Here's the drawing with two shaded views (mm, measured from the low corner). I have some questions. A direction names the side the tool comes from. Give positions to 0.01 mm unless a question says otherwise; leave off trailing zeros. Loops run counter-clockwise (first coordinate to the right, second up) from the corner with the lowest first, then second, coordinate; pieces in that order, holes last. Notation, with made-up numbers: (-32.5, 12.25) - (22.5, 12.25) arc R18 ccw to (22.5, 28.25) - close; hole circle Ø8 at (-33.5, -24). An arc over 180 degrees is marked (long way). Use a Markdown table: item, result. Add a question column.
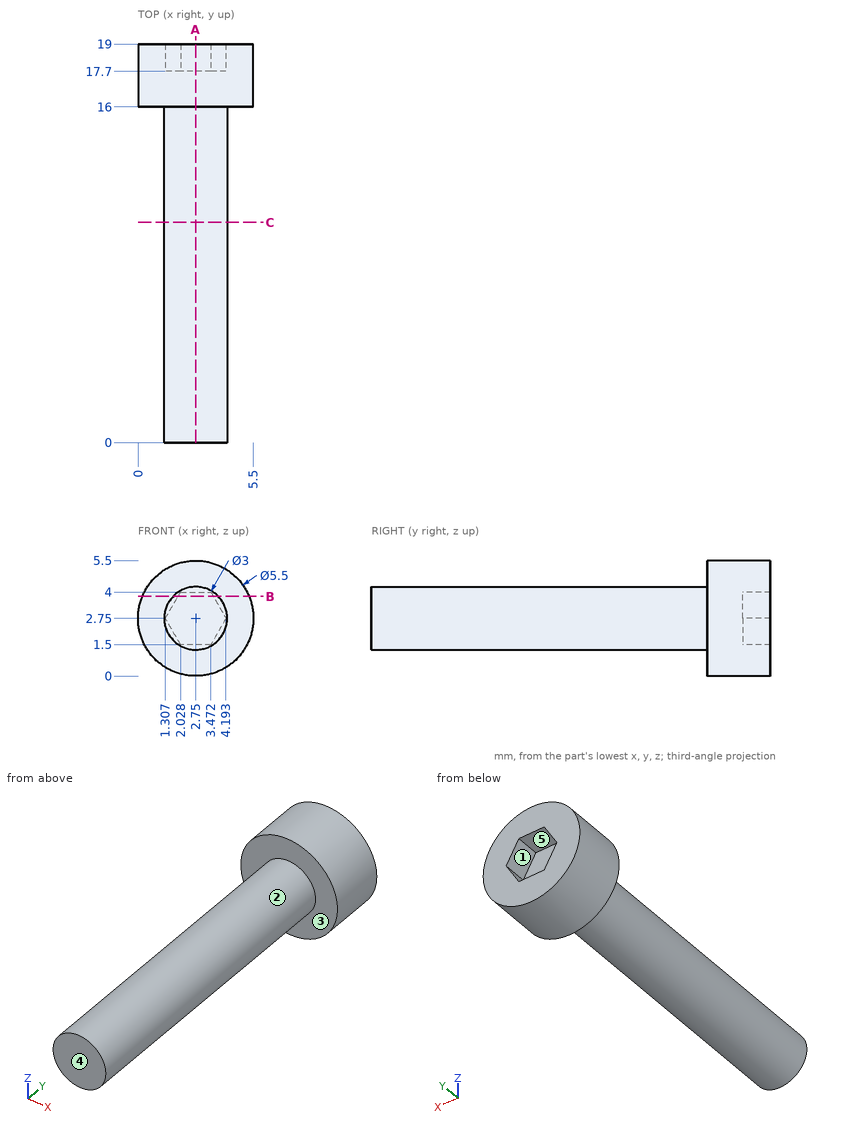
1. Suppose I cut it at B-B (z = 3.8). List the corners of the cut face in (x, y) for me.
2. If we mould it in two halves opening along X, with no side actions, what happens to the marked faces 1, 2 and 3? For each: released by +X, released by -X, zero draft, split by the parting line, or undercut.
3. Will these pins go through, and if not, where does the flat tip stop? P1, Ø1, axis at y = 2.5, z = 4.5, coming from the -X side; P2, Ø2, axis at y = 10.5, z = 3, coming from the -X side; P3, Ø3, axis at y = 5, z = 2.5, coming from the +X side.
4. Suppose I cut it at C-C (y = 10.5). List the corners of the cut face in (x, z) for me.
5. Please list where these lines run through material, in increasing order: line 1 along Y through (x, z) = (3.7, 2.3); line 2 along Y through (x, z) = (0.2, 1.85); line 3 along X through (y, z) = (5.75, 2.65). Write a range as [from, to].
6. On a 3-axis mill with a long thin cutter (end or side, diameter ignored), from which of +Z, -Z, +X, -X, +Y, -Y can I reach the whole of each face in a straight line? I mean the marked faces 4 and 5. Say none if no direction works.
7. Suppose I cut it at A-A (x = 2.75). List the corners of the cut face in (y, z) for me.
Results below:
| question | item | result |
|---|---|---|
| 1 | outline | (0.21, 16) - (1.68, 16) - (1.68, 0) - (3.82, 0) - (3.82, 16) - (5.29, 16) - (5.29, 19) - (3.59, 19) - (3.59, 17.7) - (1.91, 17.7) - (1.91, 19) - (0.21, 19) - close |
| 2 | face 1 | undercut |
| 2 | face 2 | split by the parting line |
| 2 | face 3 | zero draft |
| 3 | P1 | x = 1.92 |
| 3 | P2 | x = 1.25 |
| 3 | P3 | x = 4.25 |
| 4 | outline | circle Ø3 at (2.75, 2.75) |
| 5 | line 1 | [0, 17.7] |
| 5 | line 2 | [16, 19] |
| 5 | line 3 | [1.25, 4.25] |
| 6 | face 4 | +Z, -Z, +X, -X, -Y |
| 6 | face 5 | +Y |
| 7 | outline | (0, 1.25) - (16, 1.25) - (16, 0) - (19, 0) - (19, 1.5) - (17.7, 1.5) - (17.7, 4) - (19, 4) - (19, 5.5) - (16, 5.5) - (16, 4.25) - (0, 4.25) - close |
